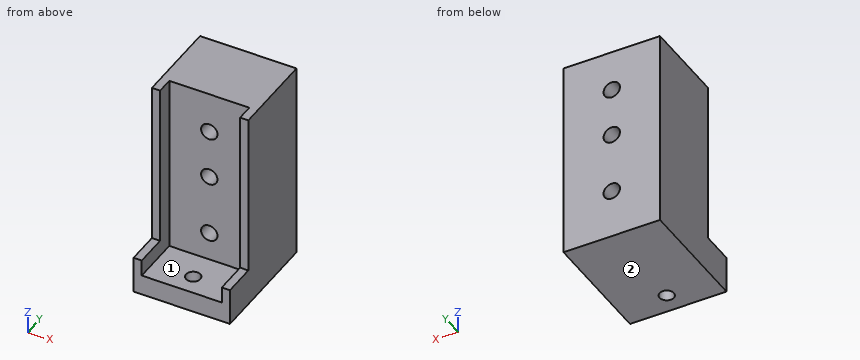
```python
from build123d import *

# Parameters (mm, degrees)
BOSS_EXTRUDE1_DEPTH = 9.75
BOSS_EXTRUDE2_DEPTH = 2
SKETCH4_R           = 2
CUT_EXTRUDE1_DEPTH  = 49.611341269
SKETCH5_R           = 1.75
CUT_EXTRUDE2_DEPTH  = 49.611341269


with BuildPart() as part:
    # Sketch2 → Boss-Extrude1 (new, symmetric)
    with BuildSketch(Plane(origin=(0, 0, 0), x_dir=(0, 0, -1), z_dir=(1, 0, 0))):
        Polygon((-44, 0), (0, 0), (0, -12), (5, -12), (5, 17), (-44, 17), align=None)
    extrude(amount=BOSS_EXTRUDE1_DEPTH, both=True)

    # Sketch3 → Boss-Extrude2 (add)
    with BuildSketch(Plane(origin=(9.75, 0, 0), x_dir=(0, 0, -1), z_dir=(1, 0, 0))):
        Polygon((-44, 17), (-44, -4), (-4, -4), (-4, -12), (5, -12), (5, 17), align=None)
    boss_extrude2 = extrude(amount=BOSS_EXTRUDE2_DEPTH)

    # Mirror1: Boss-Extrude2 across plane
    add(boss_extrude2.mirror(Plane(origin=(0, 0, 0), x_dir=(0, 0, 1), z_dir=(1, 0, 0))))

    # Sketch4 → Cut-Extrude1 (cut, through all)
    with BuildSketch(Plane.XZ):
        with Locations(Location((0, 34, 0), (0, 0, 270))):
            Circle(SKETCH4_R)
        with Locations(Location((0, 22, 0), (0, 0, 270))):
            Circle(SKETCH4_R)
        with Locations(Location((0, 7, 0), (0, 0, 270))):
            Circle(SKETCH4_R)
    extrude(amount=-CUT_EXTRUDE1_DEPTH, mode=Mode.SUBTRACT)

    # Sketch5 → Cut-Extrude2 (cut, through all)
    with BuildSketch(Plane.XY):
        with Locations((0, -7)):
            Circle(SKETCH5_R)
    extrude(amount=-CUT_EXTRUDE2_DEPTH, mode=Mode.SUBTRACT)


solid = part.part
```
Here's how the part is built. I have some questions about the finished solid (model axes, mm). Face numbers are marked on the shaded views. A direction names the side the tool comes from. Coordinates: 2 decimals unless noted, no trailing zeros. Write each loop counter-clockwise with the first axis right and the second up, starting at its lowest first coordinate (ties: lowest second). Pieces come first, ordered by that corner, then holes. Notation, with made-up numbers: (47, 62) -> (70, 62) arc R18 ccw to (70, 94) -> close; hole circle Ø8 at (-4, 78.25). An arc over 180 degrees is marked (long way). Use a Markdown table: item, result. Add a question column.
(1) If we section it at D-D, the plane y = 7.5: Write out the boundary of the cut face in (x, z), and give its area (3 significant figures).
(2) I'm going to push flat-ended pins straight in: P1, Ø1.6, axis at x = 11, y = -6, coming from the +Z side; P2, Ø5, axis at x = 0, z = 34, coming from the -Y side; P3, Ø3.5, axis at x = 0, z = 22, coming from the +Y side (3 decimals); P4, Ø3.5, axis at x = 2, y = -6, coming from the +Z side. Where does each tip first touch, or does it pass through?
(3) For the marked faces 1 and 2, which set-ups out of +Z, -Z, +X, -X, +Y, -Y let a thin tool reach every point of the face, with its end or its side?
(4) If we section it at A-A, the plane y = -7: Write out the boundary of the cut face in (x, z), and give its area (3 significant figures).
(5) Please list where these lines run through material, in increasing order: line 1 (X direction, y = -0.75, z = 32.5); line 2 (X direction, y = 4, z = 34); line 3 (Z direction, x = -0.5, y = 6).
(6) If we section it at C-C, the plane x = 0: Write out the boundary of the cut face in (y, z), and give its area (4 significant figures).
(7) If we section it at B-B, the plane z = 7: Write out the boundary of the cut face in (x, y), and give its area (4 significant figures).
Outcome:
| question | item | result |
|---|---|---|
| 1 | outline | (-11.75, -5) -> (11.75, -5) -> (11.75, 44) -> (-11.75, 44) -> close; hole circle Ø4 at (0, 7); hole circle Ø4 at (0, 22); hole circle Ø4 at (0, 34) |
| 1 | area | 1,110 mm^2 |
| 2 | P1 | stops at z = 4 |
| 2 | P2 | stops at y = 0 |
| 2 | P3 | passes through |
| 2 | P4 | stops at z = 0 |
| 3 | face 1 | +Z, -Y |
| 3 | face 2 | -Z, +X, -X, +Y, -Y |
| 4 | outline | (-11.75, -5) -> (-1.75, -5) -> (-1.75, 0) -> (-9.75, 0) -> (-9.75, 4) -> (-11.75, 4) -> close; (1.75, -5) -> (11.75, -5) -> (11.75, 4) -> (9.75, 4) -> (9.75, 0) -> (1.75, 0) -> close |
| 4 | area | 116 mm^2 |
| 5 | line 1 | x = -11.75 to -9.75, 9.75 to 11.75 |
| 5 | line 2 | x = -11.75 to -2, 2 to 11.75 |
| 5 | line 3 | z = -5 to 5.06, 8.94 to 20.06, 23.94 to 32.06, 35.94 to 44 |
| 6 | outline | (-12, -5) -> (-8.75, -5) -> (-8.75, 0) -> (-12, 0) -> close; (-5.25, -5) -> (17, -5) -> (17, 5) -> (0, 5) -> (0, 0) -> (-5.25, 0) -> close; (0, 9) -> (17, 9) -> (17, 20) -> (0, 20) -> close; (0, 24) -> (17, 24) -> (17, 32) -> (0, 32) -> close; (0, 36) -> (17, 36) -> (17, 44) -> (0, 44) -> close |
| 6 | area | 671.5 mm^2 |
| 7 | outline | (-11.75, -4) -> (-9.75, -4) -> (-9.75, 0) -> (-2, 0) -> (-2, 17) -> (-11.75, 17) -> close; (2, 0) -> (9.75, 0) -> (9.75, -4) -> (11.75, -4) -> (11.75, 17) -> (2, 17) -> close |
| 7 | area | 347.5 mm^2 |
